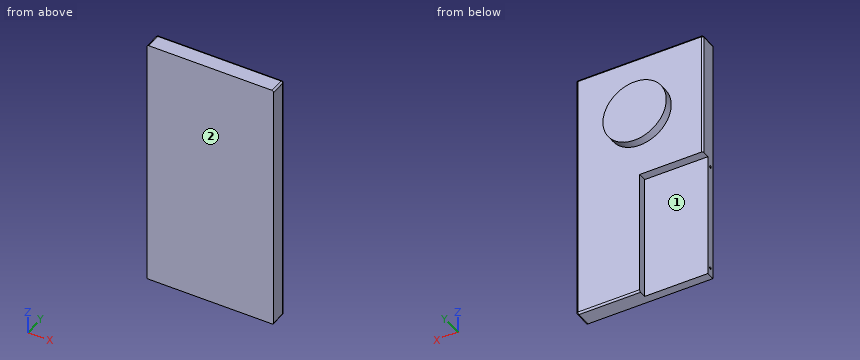
Autodesk Inventor part; units mm, degrees
ref_plane "YZ Plane" through (0, 0, 0) normal (1, 0, 0) x (0, 1, 0)
ref_plane "XZ Plane" through (0, 0, 0) normal (0, 1, 0) x (-1, 0, 0)
ref_plane "XY Plane" through (0, 0, 0) normal (0, 0, 1) x (1, 0, 0)
sketch "Sketch3" plane through (0, 0, 0) normal (0, 1, 0) x (-1, 0, 0)
  line L0 (75, 150) -> (-75, 150)
  line L1 (-75, 150) -> (-75, -150)
  line L2 (-75, -150) -> (75, -150)
  line L3 (75, -150) -> (75, 150)
  line L4 (75, 150) -> (-75, -150) construction
  line L5 (-75, 150) -> (75, -150) construction
  point P0 (0, 0)
  dimension "d7" = 150
  dimension "d8" = 300
extrude "Extrusion3" add sketch "Sketch3" along normal blind 20
sketch "Sketch4" plane through (0, 20, 0) normal (0, 1, 0) x (1, 0, 0)
  line L0 (75, 150) -> (-75, 150)
  line L1 (-75, 150) -> (0, 150)
  line L2 (0, 150) -> (0, 0)
  line L3 (0, 0) -> (-75, 0)
  line L4 (-75, 0) -> (-75, 150)
  dimension "d11" = 75
  dimension "d12" = 150
extrude "Extrusion4" cut sketch "Sketch4" against normal blind 10
sketch "Sketch5" plane through (-75, 0, -150) normal (-1, 0, 0) x (0, 0, 1)
  line L0 (0, 0) -> (300, 0)
  line L1 (0, 0) -> (0, 10)
  line L2 (150, 20) -> (150, 10)
  point P0 (150, 0)
  point P1 (10, 5)
  point P2 (140, 5)
  dimension "d15" = 5
  dimension "d16" = 5
  dimension "d17" = 10
  dimension "d18" = 10
hole "Hole1" at (-75, 5, -10) at (-75, 5, -140) direction (1, 0, 0) diameter 3 depth 5 tip angle 118
fillet "Fillet1" radius 2 4 edges at (75, 20, 0) (0, 20, 150) (37.5, 20, -150) (-75, 20, 75)
fillet "Fillet2" radius 2 6 edges at (74.4142, 19.4142, 149.4142) (75, 9, 150) (-74.4142, 19.4142, 149.4142) (-75, 9, 150) (74.4142, 19.4142, -149.4142) (75, 9, -150)
sketch "Sketch6" plane through (0, 20, 0) normal (0, 1, 0) x (1, 0, 0)
  circle A0 centre (0, -75) radius 37.5
  line L0 (-73, -150) -> (73, -150)
  line L1 (-75, 0) -> (-75, -148)
  point P0 (0, 0)
  dimension "d28" = 75
  dimension "d29" = 75
  dimension "d30" = 75
extrude "Extrusion5" add sketch "Sketch6" along normal blind 10
The model under review builds one solid part; all positions refer to its coordinate system, in mm. Face numbers are marked on the shaded views. A direction names the side the tool comes from. Round coordinates to 2 decimals unless told otherwise and drop trailing zeros. Loops run counter-clockwise (first coordinate to the right, second up) from the corner with the lowest first, then second, coordinate; pieces in that order, holes last. Notation, with made-up numbers: (-38, 72) -> (-14, 72) arc R16 cw to (-14, 83) -> close; hole circle Ø5 at (41, 37.25). An arc over 180 degrees is marked (long way). Write item = value, one per line. Start each with the question number.
Item 1: Take a section at D-D on y = 23.75. Give the boundary of the cut face in (x, z).
Item 2: To check wall thickness, follow L1, parallel to Z at x = -71.5, y = 5; L2, parallel to Y at x = -72, z = -140; L3, parallel to Y at x = -18.5, z = 133.5. State the ranges of each line that lie inside material, in increasing order.
Item 3: Take a section at C-C on x = -46. Give the boundary of the cut face in (y, z), plus the area to 3 significant figures.
Item 4: Take a section at A-A on x = 10.5. Give the boundary of the cut face in (y, z), plus the area to 3 significant figures.
Item 5: For the marked faces 1 and 2, list the 3-axis set-ups (+Z, -Z, +X, -X, +Y, -Y) from which the entire face can be reached by the end or side of a thin tool; tool diameter is ignored.
Item 6: Take a section at B-B on z = -104.5. Give the boundary of the cut face in (x, y).
Item 7: Insertion check: pin 1 (11 mm diameter, centred on x = -39, y = 16.5, fed in from -Z); pin 2 (11 mm diameter, centred on y = 16, z = -71.5, fed in from -X); pin 3 (4 mm diameter, centred on x = 34, z = -9.5, fed in from +Y); pin 4 (3 mm diameter, centred on x = -40.5, y = 23.5, fed in from -Z). Each pin has a flat end and moves straight along its axis. Give the tip position at first contact, or say it passes through.
Result:
q1.outline = circle Ø75 at (0, 75)
q2.L1 = -150 to -141.5, -138.5 to -11.5, -8.5 to 150
q2.L2 = 0 to 3.5, 6.5 to 10
q2.L3 = 0 to 20
q3.outline = (0, -150) -> (10, -150) -> (10, 0) -> (20, 0) -> (20, 148) arc R2 ccw to (18, 150) -> (0, 150) -> close
q3.area = 4,500 mm²
q4.outline = (0, -150) -> (18, -150) arc R2 ccw to (20, -148) -> (20, 39) -> (30, 39) -> (30, 111) -> (20, 111) -> (20, 148) arc R2 ccw to (18, 150) -> (0, 150) -> close
q4.area = 6,720 mm²
q5.face_1 = -Z, -X, +Y
q5.face_2 = +Z, -Z, +X, -X, -Y
q6.outline = (-75, 0) -> (75, 0) -> (75, 18) arc R2 ccw to (73, 20) -> (0, 20) -> (0, 10) -> (-75, 10) -> close
q7.pin_1 = 0
q7.pin_2 = 0
q7.pin_3 = 20
q7.pin_4 = through
